Autodesk Inventor part; units mm, degrees
ref_plane "YZ Plane" through (0, 0, 0) normal (1, 0, 0) x (0, 1, 0)
ref_plane "XZ Plane" through (0, 0, 0) normal (0, 1, 0) x (-1, 0, 0)
ref_plane "XY Plane" through (0, 0, 0) normal (0, 0, 1) x (1, 0, 0)
sketch "Sketch1" plane through (0, 0, 0) normal (0, 0, 1) x (1, 0, 0)
  line L0 (10.12, -21.6797) -> (-25.88, -21.6797)
  line L1 (-25.88, -21.6797) -> (-25.88, -12.1797)
  line L2 (-25.88, -12.1797) -> (10.12, -12.1797)
  line L3 (10.12, -12.1797) -> (10.12, -21.6797)
  line L4 (-3.88, -19.1797) -> (-11.88, -19.1797)
  line L5 (-11.88, -19.1797) -> (-11.88, -14.6797)
  line L6 (-11.88, -14.6797) -> (-3.88, -14.6797)
  line L7 (-3.88, -14.6797) -> (-3.88, -19.1797)
  line L8 (-20.9351, -12.1797) -> (-26.9351, -12.1797) construction
  point P0 (0, 0)
  point P1 (-7.88, -16.9297)
  dimension "d3" = 36
  dimension "d5" = 9.5
  dimension "d6" = 18
  dimension "d7" = 4.75
  dimension "d8" = 8
  dimension "d9" = 4.5
  dimension "d10" = 2.25
  dimension "d11" = 4
extrude "SUPPORT TABLE" add sketch "Sketch1" along normal blind 1
sketch "Sketch2" plane through (0, 0, 0) normal (0, 0, -1) x (-1, 0, 0)
  line L0 (21.9351, -13.1797) -> (21.9351, -20.6797) construction
  line L1 (21.9351, -20.6797) -> (25.9351, -20.6797) construction
  line L2 (25.9351, -20.6797) -> (25.9351, -13.1797) construction
  line L3 (25.9351, -13.1576) -> (21.9351, -13.1576) construction
  line L4 (7.838, -23.7532) -> (7.838, -10.1502) construction
  line L5 (19.882, -21.6797) -> (19.882, -12.1797)
  line L6 (19.882, -12.1797) -> (25.882, -12.1797)
  line L7 (25.882, -12.1797) -> (25.882, -21.6797)
  line L8 (25.882, -21.6797) -> (19.882, -21.6797)
  line L9 (-5.118, -13.1797) -> (-5.118, -20.6797) construction
  line L10 (-5.118, -20.6797) -> (-9.118, -20.6797) construction
  line L11 (-9.118, -20.6797) -> (-9.118, -13.1797) construction
  line L12 (-9.118, -13.1797) -> (-5.118, -13.1797) construction
  line L13 (-4.12, -21.6797) -> (-4.12, -12.1797)
  line L14 (-4.12, -12.1797) -> (-10.12, -12.1797)
  line L15 (-10.12, -12.1797) -> (-10.12, -21.6797)
  line L16 (-10.12, -21.6797) -> (-4.12, -21.6797)
  line L17 (25.88, -21.6797) -> (25.88, -12.1797) construction
  line L18 (25.88, -12.1797) -> (-10.12, -12.1797)
  point P0 (0, 0)
extrude "LEGS" add sketch "Sketch2" along normal blind 4.9
sketch "Sketch3" plane through (0, 0, 0) normal (0, 0, -1) x (-1, 0, 0)
  line L0 (25.882, -21.6797) -> (25.882, -12.1797) construction
  line L1 (19.882, -21.6797) -> (25.882, -21.6797) construction
  line L2 (19.882, -12.1797) -> (19.882, -21.6797) construction
  line L3 (19.882, -12.1797) -> (19.882, -21.6797) construction
  line L4 (19.882, -21.6797) -> (25.882, -21.6797) construction
  line L5 (25.882, -21.6797) -> (25.882, -12.1797) construction
  line L6 (25.882, -12.1797) -> (19.882, -12.1797) construction
  line L7 (-4.12, -12.1797) -> (-10.12, -12.1797) construction
  line L8 (-10.12, -12.1797) -> (-10.12, -21.6797) construction
  line L9 (-10.12, -21.6797) -> (-4.12, -21.6797) construction
  line L10 (-4.12, -21.6797) -> (-4.12, -12.1797) construction
  line L11 (24.882, -20.6797) -> (20.882, -20.6797)
  line L12 (20.882, -20.6797) -> (20.882, -13.1797)
  line L13 (20.882, -13.1797) -> (24.882, -13.1797)
  line L14 (24.882, -13.1797) -> (24.882, -20.6797)
  line L15 (7.838, -20.9409) -> (7.838, -12.9184) construction
  line L16 (-9.206, -20.6797) -> (-5.206, -20.6797)
  line L17 (-5.206, -20.6797) -> (-5.206, -13.1797)
  line L18 (-5.206, -13.1797) -> (-9.206, -13.1797)
  line L19 (-9.206, -13.1797) -> (-9.206, -20.6797)
  point P0 (0, 0)
  point P1 (7.838, -16.9297)
  point P2 (7.838, -16.9297)
  dimension "d24" = 1
  dimension "d25" = 1
  dimension "d26" = 1
  dimension "d27" = 1
extrude "PINS FOR LINEUP" add sketch "Sketch3" along normal blind 5.9
properties part number "InternalSupportBracket"
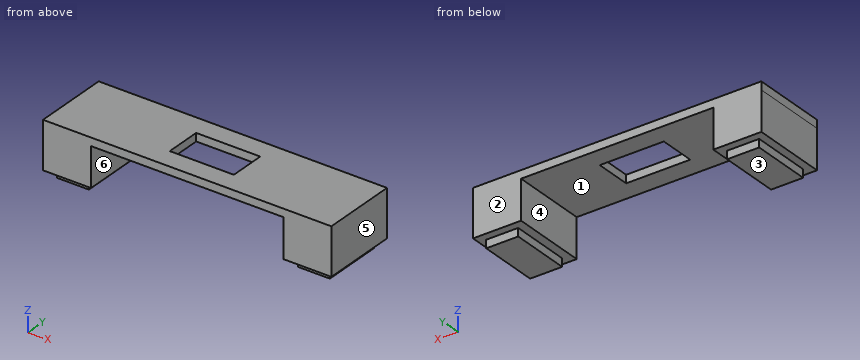
Read the model definition and answer for the solid it produces. Units are mm, in the model's axes. Face numbers are marked on the shaded views. A direction names the side the tool comes from. Give positions to 0.01 mm unless a question says otherwise; leave off trailing zeros. Loops run counter-clockwise (first coordinate to the right, second up) from the corner with the lowest first, then second, coordinate; pieces in that order, holes last.
Item 1: For the marked faces 1 and 2, determine the directions among +Z, -Z, +X, -X, +Y, -Y from which every point of the face is accessible in a straight line to the end or side of a thin tool.
Item 2: Find the intervals of material crossed by line 1 along X through (y, z) = (-20, -3.25); line 2 along X through (y, z) = (-20.25, -5.5); line 3 along Z through (x, y) = (-18, -20.25), in increasing order.
Item 3: Each of these flat-tipped pins is pushed along its axis until it touches: pin 1 Ø1.1 at (x, z) = (7, -5.5) entering from +Y; pin 2 Ø0.5 at (x, z) = (-22.5, -5.5) entering from -Y; pin 3 Ø4 at (x, y) = (-18.5, -19) entering from -Z; pin 4 Ø1.1 at (y, z) = (-16, -5) entering from -X. Where does it stop, or does it pass through?
Item 4: The part is cut by section B-B (x = -6). Write down the section's boundary in (y, z).
Item 5: The part is cut by section C-C (z = -4). Write down the section's boundary in (x, y), and give its area (3 significant figures).
Item 6: The mould has two halves that part along X. Classify the marked faces 3, 4, 5 and 6: released by +X, released by -X, zero draft, split by the parting line, or undercut.
Taken from the geometry:
1. face 1: -Z, +Y, -Y
1. face 2: +Z, -Z, +X, -X, +Y
2. line 1: x = -25.88 to -19.88, 4.12 to 10.12
2. line 2: x = -24.88 to -20.88, 5.21 to 9.21
2. line 3: z = 0 to 1
3. pin 1: stops at y = -13.18
3. pin 2: stops at y = -20.68
3. pin 3: stops at z = -4.9
3. pin 4: stops at x = -25.88
4. outline: (-21.68, 0) - (-19.18, 0) - (-19.18, 1) - (-21.68, 1) - close; (-14.68, 0) - (-12.18, 0) - (-12.18, 1) - (-14.68, 1) - close
5. outline: (-25.88, -21.68) - (-19.88, -21.68) - (-19.88, -12.18) - (-25.88, -12.18) - close; (4.12, -21.68) - (10.12, -21.68) - (10.12, -12.18) - (4.12, -12.18) - close
5. area: 114 mm2
6. face 3: zero draft
6. face 4: undercut
6. face 5: released by +X
6. face 6: undercut
